The model under review builds one solid part; all positions refer to its coordinate system, in mm. Round coordinates to 2 decimals unless told otherwise and drop trailing zeros. Write each loop counter-clockwise with the first axis right and the second up, starting at its lowest first coordinate (ties: lowest second). Pieces come first, ordered by that corner, then holes.
Item 1: Add section A-A (x = 35). Give the boundary of the cut face in (y, z), plus the area to 3 significant figures.
Item 2: Add section B-B (y = 2.65). Give the boundary of the cut face in (x, z), plus the area to 3 significant figures.
Item 3: To check wall thickness, follow L1, parallel to X at y = 1, z = 1.15; L2, parallel to Z at x = 69, y = -1.1; L3, parallel to Z at x = 58.5, y = 3.8. State the ranges of each line that lie inside material, in increasing order.
Item 4: Clearance check with flat-ended pins moving along their axes: pin 1 Ø1.2 at (x, z) = (89, 0) entering from +Y; pin 2 Ø1.6 at (x, y) = (90, 1) entering from -Z; pin 3 Ø3 at (x, y) = (31, 2.5) entering from -Z; pin 4 Ø1.6 at (x, y) = (65.5, -0.5) entering from -Z. State where each tip first meets the part, or that it passes through.
```python
from build123d import *

# Parameters (mm, degrees)
BOSS_EXTRUDE1_DEPTH = 88
SKETCH2_W           = 2
SKETCH2_H           = 2
CUT_EXTRUDE1_DEPTH  = 88
SKETCH3_W           = 1.5
SKETCH3_H           = 1.5
BOSS_EXTRUDE2_DEPTH = 3
SKETCH4_W           = 1.5
SKETCH4_H           = 1.5
BOSS_EXTRUDE3_DEPTH = 3


with BuildPart() as part:
    # Sketch1 → Boss-Extrude1 (new body)
    with BuildSketch(Plane(origin=(0, 0, 0), x_dir=(0, 0, -1), z_dir=(1, 0, 0))):
        Polygon((-1.402077652, -1.507305482), (3.597922348, -1.507305482), (3.597922348, 1.492694518), (-1.402077652, 4.381582518), align=None)
    extrude(amount=BOSS_EXTRUDE1_DEPTH)

    # Sketch2 → Cut-Extrude1 (cut)
    with BuildSketch(Plane.ZY):
        with Locations((-2.597922348, -0.507305482)):
            Rectangle(SKETCH2_W, SKETCH2_H)
    extrude(amount=-CUT_EXTRUDE1_DEPTH, mode=Mode.SUBTRACT)

    # Sketch3 → Boss-Extrude2 (add)
    with BuildSketch(Plane.ZY):
        with Locations((-0.347922348, 0.742694518)):
            Rectangle(SKETCH3_W, SKETCH3_H)
    extrude(amount=BOSS_EXTRUDE2_DEPTH)

    # Sketch4 → Boss-Extrude3 (add)
    with BuildSketch(Plane(origin=(88, 0, 0), x_dir=(0, 0, -1), z_dir=(1, 0, 0))):
        with Locations((0.347922348, 0.742694518)):
            Rectangle(SKETCH4_W, SKETCH4_H)
    extrude(amount=BOSS_EXTRUDE3_DEPTH)


solid = part.part
```
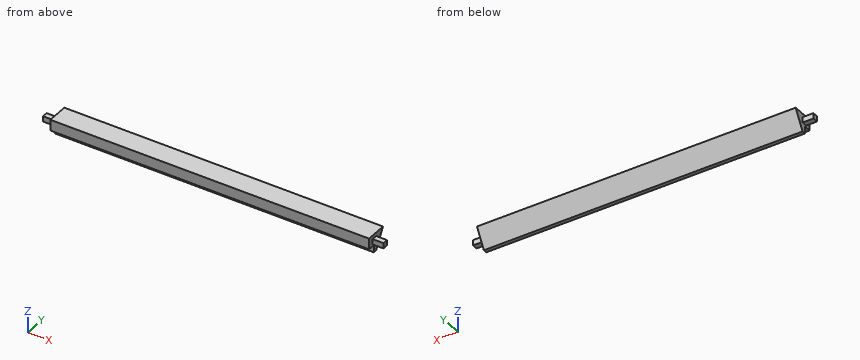
Numbers:
1. outline: (-1.51, -1.6) - (0.49, -1.6) - (0.49, -3.6) - (1.49, -3.6) - (4.38, 1.4) - (-1.51, 1.4) - close
1. area: 18.2 mm2
2. outline: (0, -1.59) - (88, -1.59) - (88, 1.4) - (0, 1.4) - close
2. area: 264 mm2
3. L1: x = 0 to 88
3. L2: z = -1.6 to 1.4
3. L3: z = 0.4 to 1.4
4. pin 1: stops at y = 1.49
4. pin 2: stops at z = -1.1
4. pin 3: stops at z = -3.6
4. pin 4: stops at z = -1.6
